```python
from build123d import *

# Parameters (mm, degrees)
SKETCH1_R           = 3.5
BOSS_EXTRUDE1_DEPTH = 3


with BuildPart() as part:
    # Sketch1 → Boss-Extrude1 (new body)
    with BuildSketch(Plane(origin=(0, 0, 0), x_dir=(0, 0, -1), z_dir=(1, 0, 0))):
        with BuildLine():
            Line((60, 60), (-60, 60))
            Line((-60, 60), (-60, -60))
            Line((-60, -60), (35, -60))
            ThreePointArc((35, -60), (52.67766953, -52.67766953), (60, -35))
            Line((60, -35), (60, 60))
        make_face()
        with Locations((40, -40)):
            Circle(SKETCH1_R, mode=Mode.SUBTRACT)
    extrude(amount=BOSS_EXTRUDE1_DEPTH)


solid = part.part
```
Check sheet for the modelled part. Datum: model origin and axes. Units: mm. Coordinates: 2 decimals unless noted, no trailing zeros. Write each loop counter-clockwise with the first axis right and the second up, starting at its lowest first coordinate (ties: lowest second). Pieces come first, ordered by that corner, then holes. Notation, with made-up numbers: M 57,-18.5 L 80,-18.5 A18 ccw 80,2.5 Z; hole C -27,17.25 d11. An arc over 180 degrees is marked long. Use one line per item in the form item = value.
Item 1: Release check for a two-part mould opening along Y. For faces 1 (the face through (1.479, -37.635, -37.42)), 2 (the face through (1, 1, 60)), 3 (the face through (1.479, -52.871, -52.482)) record: pulls with the +Y half, pulls with the -Y half, needs draft (parallel to the pull), parting line crosses it, or undercut.
Answer below:
face_1 = undercut
face_2 = needs draft
face_3 = pulls with the -Y half
Item 2: Material ranges on L1, parallel to Z at x = 2.1, y = -38; L2, parallel to Y at x = 0.95, z = -40; L3, parallel to Z at x = 0.4, y = -53.5, recorded low to high. Write a range as from..to.
Answer below:
L1 = -59.82..-42.87, -37.13..60
L2 = -59.49..-43.5, -36.5..60
L3 = -51.82..60
Item 3: Gauge pin test, flat end, axial feed: pin 1 Ø2 at (y, z) = (-31, -19.5) entering from -X. Record the tip position at first contact, or that the pin passes through.
Answer below:
pin_1 = 0
Item 4: Sectioned sample at A-A, the plane z = -40. Record the cut outline in (x, y), and give its area (3 significant figures).
Answer below:
outline = M 0,-59.49 L 3,-59.49 L 3,-43.5 L 0,-43.5 Z; M 0,-36.5 L 3,-36.5 L 3,60 L 0,60 Z
area = 337 mm^2
